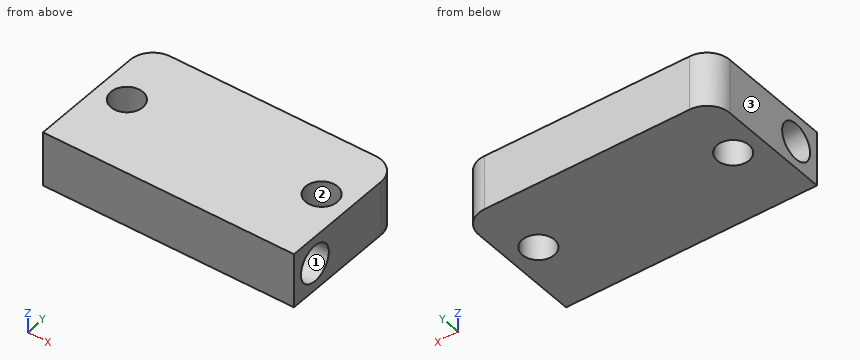
Autodesk Inventor part; units mm, degrees
ref_plane "YZ Plane" through (0, 0, 0) normal (1, 0, 0) x (0, 1, 0)
ref_plane "XZ Plane" through (0, 0, 0) normal (0, 1, 0) x (-1, 0, 0)
ref_plane "XY Plane" through (0, 0, 0) normal (0, 0, 1) x (1, 0, 0)
sketch "Boceto1" plane through (0, 0, 0) normal (0, 0, 1) x (1, 0, 0)
  line L0 (0, 0) -> (55, 0)
  line L1 (55, 0) -> (55, 20)
  line L2 (55, 20) -> (0, 20)
  line L3 (0, 20) -> (0, 0)
  circle A0 centre (6.165, 6) radius 3.5
  line L4 (27.5, 20) -> (27.5, 0)
  circle A1 centre (48.835, 6) radius 3.5
  dimension "d0" = 7
  dimension "d1" = 55
  dimension "d3" = 20
  dimension "d23" = 42.67
  dimension "d32" = 6
extrude "Extrusión1" add sketch "Boceto1" along normal blind 12
fillet "Empalme1" radius 5 2 edges at (55, 20, 6) (0, 20, 6)
sketch "Boceto7" plane through (0, 0, 0) normal (0, -1, 0) x (1, 0, 0)
  line L0 (0, 0) -> (0, 12)
  line L1 (0, 12) -> (55, 12)
  line L2 (0, 0) -> (55, 0)
  line L3 (55, 0) -> (55, 12)
  line L4 (55, 12) -> (0, 12)
  line L5 (0, 12) -> (0, 0)
extrude "Extrusión5" add sketch "Boceto7" along normal blind 10
sketch "Boceto8" plane through (55, 15, 12) normal (1, 0, 0) x (0, 0, -1)
  circle A0 centre (6, -19) radius 4
  line L0 (12, -25) -> (0, -25)
  line L1 (12, 0) -> (12, -25)
  point P0 (12, -15)
  point P1 (6, -25)
  dimension "d26" = 8
  dimension "d27" = 6
extrude "Extrusión6" cut sketch "Boceto8" against normal blind 55
properties part number "SoporteDerecha"
Work out the finished part from the listing and answer in its coordinate system (mm). Face numbers are marked on the shaded views. Give positions to 0.01 mm unless a question says otherwise; leave off trailing zeros. Write each loop counter-clockwise with the first axis right and the second up, starting at its lowest first coordinate (ties: lowest second). Pieces come first, ordered by that corner, then holes.
Q1. The part is cut by section B-B on y = 6. Give the vertices of the cut face in (x, z) (3 decimals).
Answer:
outline: (0, 0) - (2.665, 0) - (2.665, 12) - (0, 12) - close; (9.665, 0) - (45.335, 0) - (45.335, 12) - (9.665, 12) - close; (52.335, 0) - (55, 0) - (55, 12) - (52.335, 12) - close
Q2. For a pull along X with two mould halves and no side action, classify the marked faces 1, 2 and 3 as released by +X, released by -X, zero draft, split by the parting line, or undercut.
Answer:
face 1: zero draft
face 2: undercut
face 3: released by -X
Q3. The part is cut by section A-A on z = 6. Give the vertices of the cut face in (x, y) (3 decimals), and give its area (3 significant figures).
Answer:
outline: (0, -10) - (55, -10) - (55, -8) - (0, -8) - close; (0, 0) - (55, 0) - (55, 15) arc R5 ccw to (50, 20) - (5, 20) arc R5 ccw to (0, 15) - close; hole circle Ø7 at (6.165, 6); hole circle Ø7 at (48.835, 6)
area: 1,120 mm2
Q4. Straight lines are drawn through the part: L1, parallel to Y at x = 42, z = 6; L2, parallel to Y at x = 8, z = 3.5; L3, parallel to Y at x = 52, z = 4.75. For each, find the intervals that lie inside material, in ascending order.
Answer:
L1: y = -10 to -8, 0 to 20
L2: y = -10 to -7.12, -0.88 to 3.02, 8.98 to 20
L3: y = -10 to -7.8, -0.2 to 4.51, 7.49 to 19.58
Q5. Given pin 1 (6.5 mm diameter, centred on x = 48.835, y = 6, fed in from +Z), flat-ended and moving along its own axis, determine where the tip first touches the part or whether it passes through.
Answer:
pin 1: passes through
Q6. The part is cut by section C-C on x = 49. Give the vertices of the cut face in (y, z).
Answer:
outline: (-10, 0) - (2.5, 0) - (2.5, 12) - (-10, 12) - close; (9.5, 0) - (20, 0) - (20, 12) - (9.5, 12) - close; hole circle Ø8 at (-4, 6)
Q7. The part is cut by section D-D on y = -4. Give the vertices of the cut face in (x, z).
Answer:
outline: (0, 0) - (55, 0) - (55, 2) - (0, 2) - close; (0, 10) - (55, 10) - (55, 12) - (0, 12) - close
